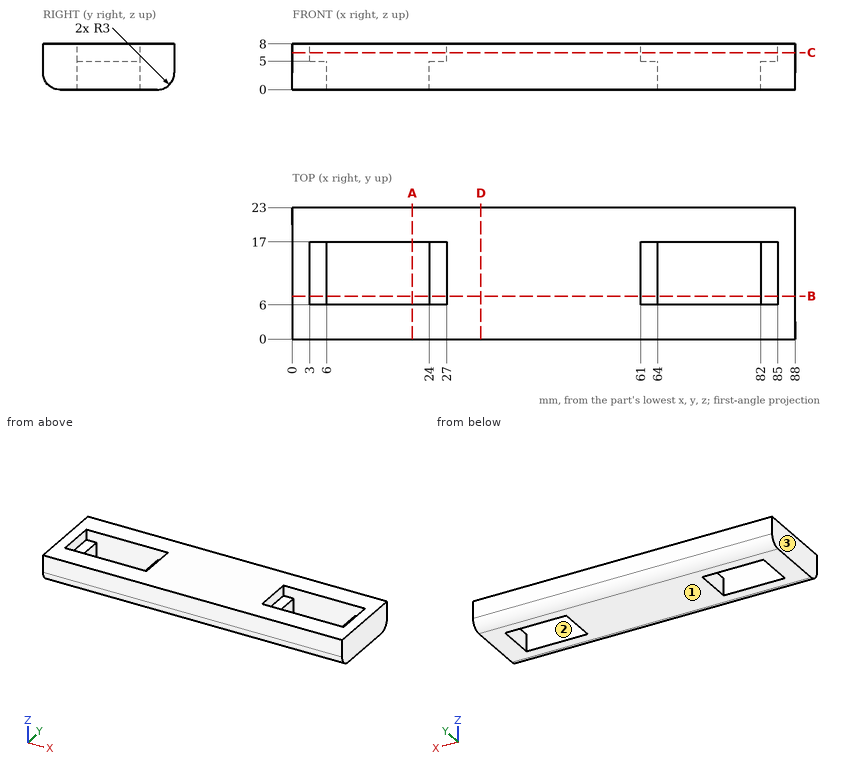
Study the drawing (mm; zero at the part's minimum x, y, z) and answer. Coordinates: 2 decimals unless noted, no trailing zeros. Loops run counter-clockwise (first coordinate to the right, second up) from the corner with the lowest first, then second, coordinate; pieces in that order, holes last. Notation, with made-up numbers: M -25.5,21.5 L -14.5,21.5 A36 ccw -14.5,57.5 Z; hole C 4.25,-7 d1. An arc over 180 degrees is marked long. Answer in a Markdown table with one row per item.
1) Find section C-C (z = 6.5). Determine the outline of the cut face in (x, y).
Answers below:
| item | result |
|---|---|
| outline | M 0,0 L 88,0 L 88,23 L 0,23 Z; hole M 3,6 L 27,6 L 27,17 L 3,17 Z; hole M 61,6 L 85,6 L 85,17 L 61,17 Z |
2) Find the intervals of material crossed by probe 1 along X at (y, z) = (10.75, 7.5); probe 2 along X at (y, z) = (12.5, 4.75); probe 3 along Y at (x, z) = (17, 4.5), in increasing order.
Answers below:
| item | result |
|---|---|
| probe 1 | 0 to 3, 27 to 61, 85 to 88 |
| probe 2 | 0 to 6, 24 to 64, 82 to 88 |
| probe 3 | 0 to 6, 17 to 23 |
3) Find section A-A (x = 21). Determine the outline of the cut face in (y, z), then the cut area to 3 significant figures.
Answers below:
| item | result |
|---|---|
| outline | M 0,3 A3 ccw 3,0 L 6,0 L 6,8 L 0,8 Z; M 17,0 L 20,0 A3 ccw 23,3 L 23,8 L 17,8 Z |
| area | 92.1 mm^2 |
4) Find section D-D (x = 33). Determine the outline of the cut face in (y, z), then the cut area to 3 significant figures.
Answers below:
| item | result |
|---|---|
| outline | M 0,3 A3 ccw 3,0 L 20,0 A3 ccw 23,3 L 23,8 L 0,8 Z |
| area | 180 mm^2 |
5) Given pin 1 (2.5 mm diameter, centred on x = 25, y = 13.5, fed in from +Z), flat-ended and moving along its own axis, determine where the tip first touches the part or whether it passes through.
Answers below:
| item | result |
|---|---|
| pin 1 | z = 5 |
6) Find section B-B (y = 7.5). Determine the outline of the cut face in (x, z).
Answers below:
| item | result |
|---|---|
| outline | M 0,0 L 6,0 L 6,5 L 3,5 L 3,8 L 0,8 Z; M 24,0 L 64,0 L 64,5 L 61,5 L 61,8 L 27,8 L 27,5 L 24,5 Z; M 82,0 L 88,0 L 88,8 L 85,8 L 85,5 L 82,5 Z |
7) Determine the mould class of the marked faces 1, 2 and 3 for opening direction X: released by +X, released by -X, zero draft, split by the parting line, or undercut.
Answers below:
| item | result |
|---|---|
| face 1 | zero draft |
| face 2 | undercut |
| face 3 | released by -X |
